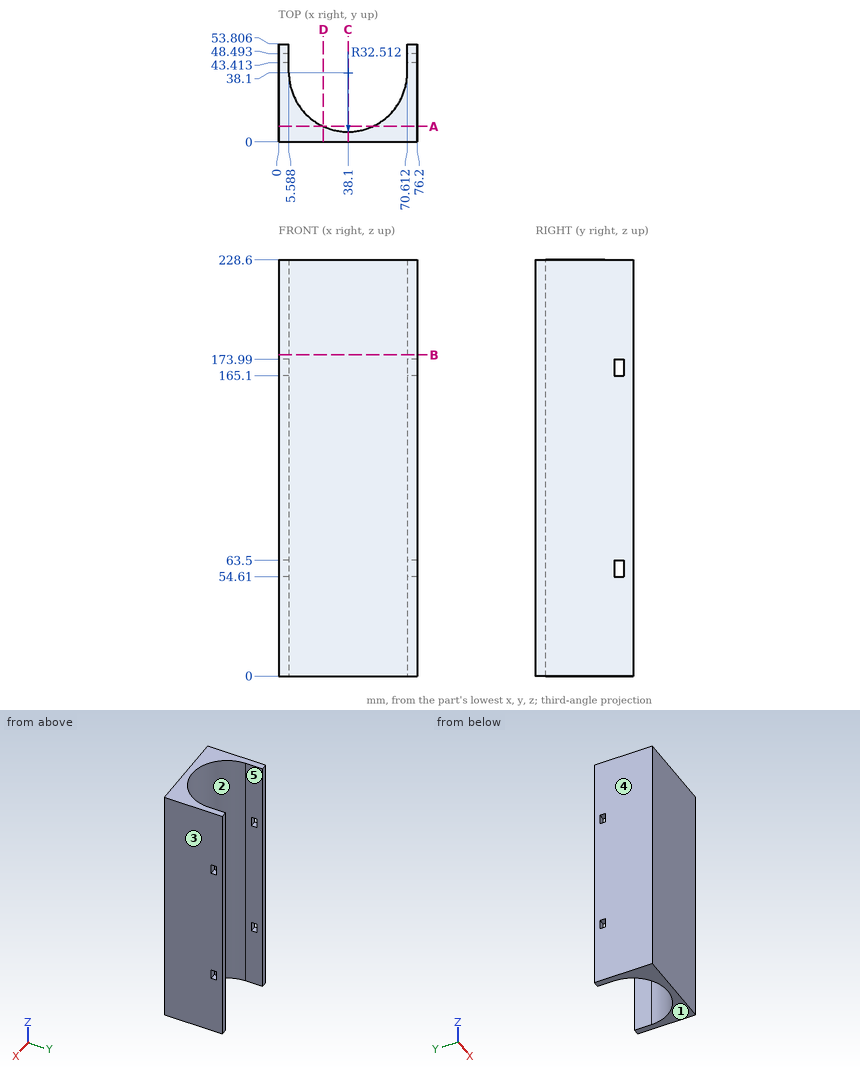
Design review of the part shown in the three views and the two pictorial views. Dimensions are in mm from the part's minimum x, y and z. A direction names the side the tool comes from. Round coordinates to 2 decimals unless told otherwise and drop trailing zeros. Loops run counter-clockwise (first coordinate to the right, second up) from the corner with the lowest first, then second, coordinate; pieces in that order, holes last. Notation, with made-up numbers: M 50,49.5 L 82,49.5 A24 cw 82,72.5 Z; hole C 61,10.5 d7. An arc over 180 degrees is marked long. Answer as a JSON object with one key per item and string values.
Item 1: We need section A-A, the plane y = 8.5. State the section outline as (x, z) points, and give its area (3 significant figures).
Check sheet entries:
{"outline": "M 0,0 L 24.65,0 L 24.65,228.6 L 0,228.6 Z; M 51.55,0 L 76.2,0 L 76.2,228.6 L 51.55,228.6 Z", "area": "11,300 mm2"}
Item 2: Tool access review of the marked faces 4 and 5: name each direction out of +Z, -Z, +X, -X, +Y, -Y from which nothing blocks a thin tool from reaching the whole face with its end or side.
Check sheet entries:
{"face 4": "+Z, -Z, -X, +Y, -Y", "face 5": "+Z, -Z, +Y"}
Item 3: Clearance check with flat-ended pins moving along their axes: P1, Ø6, axis at x = 62.5, z = 51, coming from the +Y side; P2, Ø10, axis at x = 50, z = 53.5, coming from the -Y side. State where each tip first meets the part, or that it passes through.
Check sheet entries:
{"P1": "y = 20.6", "P2": "y = 0"}
Item 4: We need section C-C, the plane x = 38.1. State the section outline as (y, z) points, and give its area (3 significant figures).
Check sheet entries:
{"outline": "M 0,0 L 5.59,0 L 5.59,228.6 L 0,228.6 Z", "area": "1,280 mm2"}
Item 5: We need section B-B, the plane z = 176.5. State the section outline as (x, y) points (1 decimal), and give its area (3 significant figures).
Check sheet entries:
{"outline": "M 0,0 L 76.2,0 L 76.2,53.8 L 70.6,53.8 L 70.6,38.1 A32.5 cw 5.6,38.1 L 5.6,53.8 L 0,53.8 Z", "area": "1,420 mm2"}
Item 6: The part is to be moulded in two halves that separate along X. For the marked faces 1, 2 and 3, say which applies: +X half, -X half, draft (parallel to the pull), parting line (faces both ways), or undercut.
Check sheet entries:
{"face 1": "draft", "face 2": "undercut", "face 3": "+X half"}
Item 7: We need section D-D, the plane x = 24.5. State the section outline as (y, z) points, and give its area (3 significant figures).
Check sheet entries:
{"outline": "M 0,0 L 8.57,0 L 8.57,228.6 L 0,228.6 Z", "area": "1,960 mm2"}
Item 8: For line 1 along X through (y, z) = (15, 72.5); line 2 along X through (y, z) = (24.5, 106.5); line 3 along Y through (x, z) = (31.5, 175) (1 decimal), list the stretches that pass through material, from the lowest coordinate up.
Check sheet entries:
{"line 1": "0 to 15.22, 60.98 to 76.2", "line 2": "0 to 8.57, 67.63 to 76.2", "line 3": "0 to 6.3"}
